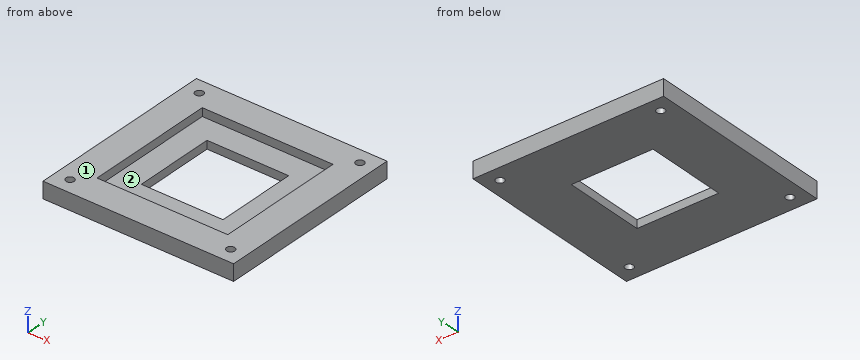
from build123d import *

# Parameters (mm, degrees)
SKETCH_W        = 35
SKETCH_H        = 35
PAD_DEPTH       = 3
SKETCH001_W     = 24
SKETCH001_H     = 24
POCKET_DEPTH    = 1.5
SKETCH002_W     = 15
SKETCH002_H     = 15
POCKET001_DEPTH = 1.5
SKETCH003_R     = 0.75
POCKET002_DEPTH = 3


with BuildPart() as part:
    # Sketch → Pad (new body)
    with BuildSketch(Plane.XY):
        with Locations((17.5, 17.5)):
            Rectangle(SKETCH_W, SKETCH_H)
    extrude(amount=PAD_DEPTH)

    # Sketch001 (on Face6 of Pad) → Pocket (cut)
    with BuildSketch(Plane.XY.offset(3)):
        with Locations((17.5, 17.5)):
            Rectangle(SKETCH001_W, SKETCH001_H)
    extrude(amount=-POCKET_DEPTH, mode=Mode.SUBTRACT)

    # Sketch002 (on Face11 of Pocket) → Pocket001 (cut)
    with BuildSketch(Plane.XY.offset(1.5)):
        with Locations((17.5, 17.5)):
            Rectangle(SKETCH002_W, SKETCH002_H)
    extrude(amount=-POCKET001_DEPTH, mode=Mode.SUBTRACT)

    # Sketch003 (on Face5 of Pocket001) → Pocket002 (cut)
    with BuildSketch(Plane.XY.offset(3)):
        with Locations((2.75, 32.25)):
            Circle(SKETCH003_R)
        with Locations((32.25, 32.25)):
            Circle(SKETCH003_R)
        with Locations((32.25, 2.75)):
            Circle(SKETCH003_R)
        with Locations((2.75, 2.75)):
            Circle(SKETCH003_R)
    extrude(amount=-POCKET002_DEPTH, mode=Mode.SUBTRACT)


solid = part.part
Verification items for the finished model (mm, model axes). Face numbers are marked on the shaded views. Coordinates: 2 decimals unless noted, no trailing zeros. Order: outer loops, then holes, each group sorted by start corner. A loop starts at its lowest first (then second) coordinate and runs counter-clockwise, first axis right, second up. Notation, with made-up numbers: (35, 65) -> (66, 65) arc R34 cw to (66, 101) -> close; hole circle Ø6 at (9, 24.25). An arc over 180 degrees is marked (long way). Put each result on its own line as item: value. Start each with the question number.
1. Cross-section at B-B, the plane y = 24. Record the boundary of the cut face in (x, z), then the cut area to 3 significant figures.
2. Mould release check, pull along X, two halves, no side actions. Record for the marked faces 1 and 2: released by +X, released by -X, zero draft, split by the parting line, or undercut.
3. Cross-section at A-A, the plane x = 32.25. Record the boundary of the cut face in (y, z), then the cut area to 3 significant figures.
4. Material ranges on L1, parallel to Y at x = 2.75, z = 1.7; L2, parallel to Y at x = 15, z = 1.7, recorded low to high. Write a range as [from, to].
5. Go/stop test with a flat-tipped pin: pin 1 Ø12 at (x, y) = (23, 15.5) entering from +Z. Record where the tip stops, or that it passes through.
6. Cross-section at D-D, the plane z = 1.1. Record the boundary of the cut face in (x, y).
Computed:
1. outline: (0, 0) -> (10, 0) -> (10, 1.5) -> (5.5, 1.5) -> (5.5, 3) -> (0, 3) -> close; (25, 0) -> (35, 0) -> (35, 3) -> (29.5, 3) -> (29.5, 1.5) -> (25, 1.5) -> close
1. area: 46.5 mm2
2. face 1: zero draft
2. face 2: undercut
3. outline: (0, 0) -> (2, 0) -> (2, 3) -> (0, 3) -> close; (3.5, 0) -> (31.5, 0) -> (31.5, 3) -> (3.5, 3) -> close; (33, 0) -> (35, 0) -> (35, 3) -> (33, 3) -> close
3. area: 96.0 mm2
4. L1: [0, 2], [3.5, 31.5], [33, 35]
4. L2: [0, 5.5], [29.5, 35]
5. pin 1: z = 1.5
6. outline: (0, 0) -> (35, 0) -> (35, 35) -> (0, 35) -> close; hole circle Ø1.5 at (2.75, 2.75); hole circle Ø1.5 at (2.75, 32.25); hole (10, 10) -> (25, 10) -> (25, 25) -> (10, 25) -> close; hole circle Ø1.5 at (32.25, 2.75); hole circle Ø1.5 at (32.25, 32.25)
